```python
from build123d import *

# Parameters (mm, degrees)
BOSS_EXTRUDE1_DEPTH = 15.24


with BuildPart() as part:
    # Sketch1 → Revolve1 (revolve)
    with BuildSketch(Plane.XY):
        with BuildLine():
            Line((0, 0), (-101.6, 0))
            Line((-101.6, 0), (-101.6, 25.4))
            Line((-101.6, 25.4), (-19.05, 25.4))
            ThreePointArc((-19.05, 25.4), (-12.7, 19.05), (-6.35, 25.4))
            Line((-6.35, 25.4), (0, 25.4))
            Line((0, 25.4), (0, 12.7))
            Line((0, 12.7), (88.9, 12.7))
            Line((88.9, 12.7), (88.9, 0))
            Line((88.9, 0), (0, 0))
        make_face()
    revolve(axis=Axis((0, 0, 0), (-1, 0, 0)))

    # Sketch2 → Boss-Extrude1 (add)
    with BuildSketch(Plane(origin=(88.9, 0, 0), x_dir=(0, 0, -1), z_dir=(1, 0, 0))):
        Polygon((8.288184077, -7.230041819), (10.405491924, 3.562757053), (2.117307847, 10.792798872), (-8.288184077, 7.230041819), (-10.405491924, -3.562757053), (-2.117307847, -10.792798872), align=None)
    extrude(amount=BOSS_EXTRUDE1_DEPTH)


solid = part.part
```
Verification items for the finished model (mm, model axes). A direction names the side the tool comes from. Give positions to 0.01 mm unless a question says otherwise; leave off trailing zeros. Loops run counter-clockwise (first coordinate to the right, second up) from the corner with the lowest first, then second, coordinate; pieces in that order, holes last.
1. Go/stop test with flat-tipped pins: pin 1 Ø8 at (x, y) = (51.5, -6) entering from -Z; pin 2 Ø8 at (x, y) = (82, -17.5) entering from -Z; pin 3 Ø3 at (x, y) = (68, 2.5) entering from +Z; pin 4 Ø8 at (x, y) = (-26.5, -13) entering from -Z. Record where each tip stops, or that it passes through.
2. Section check B-B, the plane y = 0. Enter the section's corners in (x, z), then the cut area to 3 significant figures.
3. Thickness scan on line 1 (Y direction, x = -65.5, z = 0.5); line 2 (Z direction, x = -4, y = -22); line 3 (X direction, y = -21.5, z = -11). Record the ranges inside material, lowest first.
4. Section check D-D, the plane x = 25. Enter the section's corners in (y, z).
5. Set-up check for faces 1 (the flat face through (96.413, -9.036, -3.013)), 2 (the flat face through (96.413, -7.127, 6.319)), 3 (the flat face through (96.41, 1.91, 9.33)), 4 (the flat face through (0, 5, -12)): record each of +Z, -Z, +X, -X, +Y, -Y from which the full face is reachable in a straight line by a thin tool's end or side.
6. Section check C-C, the plane z = 0. Enter the section's corners in (x, y).
7. Section check A-A, the plane x = -30. Enter the section's corners in (y, z).
Geometry says:
1. pin 1: stops at z = -12.54
1. pin 2: passes through
1. pin 3: stops at z = 12.66
1. pin 4: stops at z = -23.75
2. outline: (-101.6, -25.4) - (-19.05, -25.4) arc R6.35 cw to (-6.35, -25.4) - (0, -25.4) - (0, -12.7) - (88.9, -12.7) - (88.9, -9.71) - (104.14, -9.71) - (104.14, 9.71) - (88.9, 9.71) - (88.9, 12.7) - (0, 12.7) - (0, 25.4) - (-6.35, 25.4) arc R6.35 cw to (-19.05, 25.4) - (-101.6, 25.4) - close
2. area: 7,590 mm2
3. line 1: y = -25.4 to 25.4
3. line 2: z = -12.69 to 12.69
3. line 3: x = -101.6 to -18.93, -6.47 to 0
4. outline: circle Ø25.4 at (0, 0)
5. face 1: -Z, +X, -Y
5. face 2: +Z, +X, -Y
5. face 3: +Z, +X, +Y
5. face 4: +X
6. outline: (-101.6, -25.4) - (-19.05, -25.4) arc R6.35 cw to (-6.35, -25.4) - (0, -25.4) - (0, -12.7) - (88.9, -12.7) - (88.9, -10.07) - (104.14, -10.07) - (104.14, 10.07) - (88.9, 10.07) - (88.9, 12.7) - (0, 12.7) - (0, 25.4) - (-6.35, 25.4) arc R6.35 cw to (-19.05, 25.4) - (-101.6, 25.4) - close
7. outline: circle Ø50.8 at (0, 0)
